The drawing under review shows one solid part. Ordinate dimensions are in mm from its lowest x, y, z. Coordinates: 2 decimals unless noted, no trailing zeros. Loops run counter-clockwise (first coordinate to the right, second up) from the corner with the lowest first, then second, coordinate; pieces in that order, holes last. Notation, with made-up numbers: (26, 89) -> (45, 89) arc R19 cw to (45, 98) -> close; hole circle Ø11 at (44.25, 51.5). An arc over 180 degrees is marked (long way). Use a Markdown table: item, result.
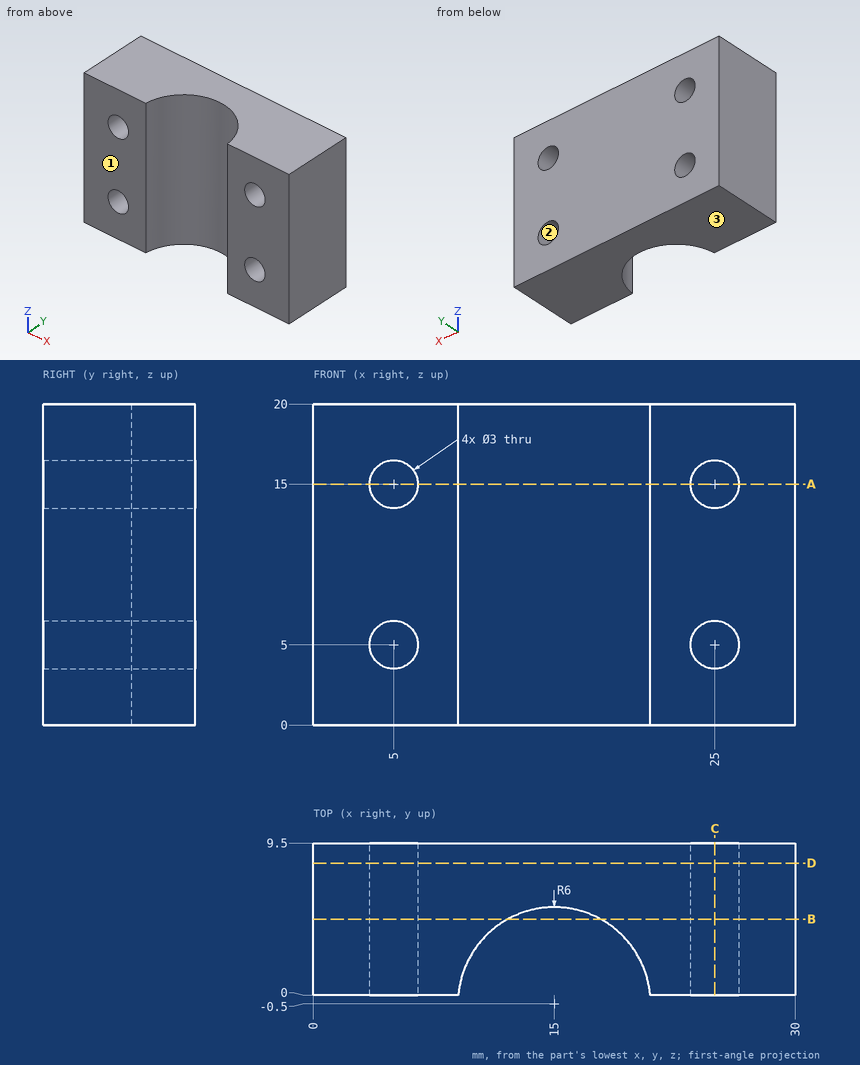
(1) Mouldability with a two-part tool opening along Z and no side actions: class the marked faces 1, 2 and 3 as pulls with the +Z half, pulls with the -Z half, needs draft (parallel to the pull), parting line crosses it, or undercut.
Found:
| item | result |
|---|---|
| face 1 | needs draft |
| face 2 | undercut |
| face 3 | pulls with the -Z half |
(2) Take a section at A-A on z = 15. Write out the cut boundary in (x, y), plus the area to 3 significant figures.
Found:
| item | result |
|---|---|
| outline | (0, 0) -> (3.5, 0) -> (3.5, 9.5) -> (0, 9.5) -> close; (6.5, 0) -> (9.02, 0) arc R6 cw to (20.98, 0) -> (23.5, 0) -> (23.5, 9.5) -> (6.5, 9.5) -> close; (26.5, 0) -> (30, 0) -> (30, 9.5) -> (26.5, 9.5) -> close |
| area | 177 mm^2 |
(3) For line 1 along Z through (x, y) = (25, 5.75); line 2 along X through (y, z) = (6, 15); line 3 along X through (y, z) = (3.5, 5), list the stretches that pass through material, from the lowest coordinate up.
Found:
| item | result |
|---|---|
| line 1 | z = 0 to 3.5, 6.5 to 13.5, 16.5 to 20 |
| line 2 | x = 0 to 3.5, 6.5 to 23.5, 26.5 to 30 |
| line 3 | x = 0 to 3.5, 6.5 to 10.53, 19.47 to 23.5, 26.5 to 30 |
(4) Take a section at C-C on x = 25. Write out the cut boundary in (y, z).
Found:
| item | result |
|---|---|
| outline | (0, 0) -> (9.5, 0) -> (9.5, 3.5) -> (0, 3.5) -> close; (0, 6.5) -> (9.5, 6.5) -> (9.5, 13.5) -> (0, 13.5) -> close; (0, 16.5) -> (9.5, 16.5) -> (9.5, 20) -> (0, 20) -> close |
(5) Take a section at B-B on y = 4.75. Write out the cut boundary in (x, z), plus the area to 3 significant figures.
Found:
| item | result |
|---|---|
| outline | (0, 0) -> (12.1, 0) -> (12.1, 20) -> (0, 20) -> close; (17.9, 0) -> (30, 0) -> (30, 20) -> (17.9, 20) -> close; hole circle Ø3 at (5, 5); hole circle Ø3 at (5, 15); hole circle Ø3 at (25, 5); hole circle Ø3 at (25, 15) |
| area | 456 mm^2 |
(6) Take a section at D-D on y = 8.25. Write out the cut boundary in (x, z).
Found:
| item | result |
|---|---|
| outline | (0, 0) -> (30, 0) -> (30, 20) -> (0, 20) -> close; hole circle Ø3 at (5, 5); hole circle Ø3 at (5, 15); hole circle Ø3 at (25, 5); hole circle Ø3 at (25, 15) |
